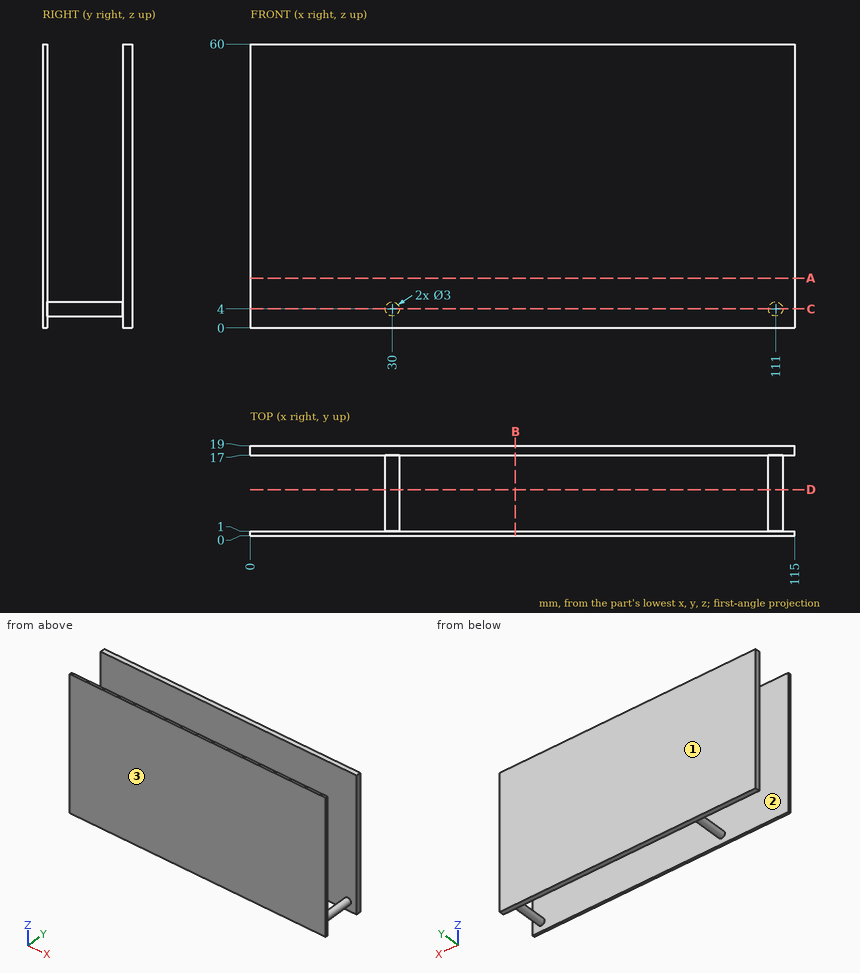
Study the drawing (mm; zero at the part's minimum x, y, z) and answer. Give positions to 0.01 mm unless a question says otherwise; leave off trailing zeros. Order: outer loops, then holes, each group sorted by start corner. A loop starts at its lowest first (then second) coordinate and runs counter-clockwise, first axis right, second up.
1) Find section A-A on z = 10.5. Write down the section's boundary in (x, y).
Reported:
outline: (0, 0) - (115, 0) - (115, 1) - (0, 1) - close; (0, 17) - (115, 17) - (115, 19) - (0, 19) - close
2) Find section C-C on z = 4. Write down the section's boundary in (x, y).
Reported:
outline: (0, 0) - (115, 0) - (115, 1) - (112.5, 1) - (112.5, 17) - (115, 17) - (115, 19) - (0, 19) - (0, 17) - (28.5, 17) - (28.5, 1) - (0, 1) - close; hole (31.5, 1) - (109.5, 1) - (109.5, 17) - (31.5, 17) - close
3) Determine the mould class of the marked faces 1, 2 and 3 for opening direction Y: pulls with the +Y half, pulls with the -Y half, needs draft (parallel to the pull), parting line crosses it, or undercut.
Reported:
face 1: pulls with the +Y half
face 2: undercut
face 3: pulls with the -Y half
4) Find section B-B on x = 56. Write down the section's boundary in (y, z).
Reported:
outline: (0, 0) - (1, 0) - (1, 60) - (0, 60) - close; (17, 0) - (19, 0) - (19, 60) - (17, 60) - close
5) Consider line 1 along Y through (x, z) = (88, 26); line 2 along X through (y, z) = (4.5, 3). Determine where each line is inside the solid, lowest interval first.
Reported:
line 1: y = 0 to 1, 17 to 19
line 2: x = 28.88 to 31.12, 109.88 to 112.12
6) Find section D-D on y = 9.75. Write down the section's boundary in (x, z), then the cut area to 3 significant figures.
Reported:
outline: circle Ø3 at (30, 4); circle Ø3 at (111, 4)
area: 14.1 mm2
